```python
from build123d import *

# Parameters (mm, degrees)
SKETCH1_R           = 2.345368149
BOSS_EXTRUDE1_DEPTH = 8.89
SKETCH2_R           = 9.131634977
BOSS_EXTRUDE2_DEPTH = 10
SKETCH3_R           = 7.205640658
CUT_EXTRUDE1_DEPTH  = 2.54
FILLET1_R           = 2.54
FILLET2_R           = 2.54


# Some blends are built 0.0001 mm under size
with BuildPart() as part:
    # Sketch1 → Boss-Extrude1 (new body)
    with BuildSketch(Plane.XY):
        with Locations((21.750777604, -13.836740686)):
            Circle(SKETCH1_R)
    extrude(amount=BOSS_EXTRUDE1_DEPTH)

    # Sketch2 → Boss-Extrude2 (add)
    with BuildSketch(Plane.XY.offset(8.89)):
        with Locations((21.750777604, -13.836740686)):
            Circle(SKETCH2_R)
    extrude(amount=BOSS_EXTRUDE2_DEPTH)

    # Sketch3 → Cut-Extrude1 (cut)
    with BuildSketch(Plane.XY.offset(18.89)):
        with Locations((21.750777604, -13.836740686)):
            Circle(SKETCH3_R)
    extrude(amount=-CUT_EXTRUDE1_DEPTH, mode=Mode.SUBTRACT)

    # Fillet1
    fillet1_edges = [part.edges().sort_by_distance(p)[0] for p in [
        (14.545136946, -13.836740686, 16.35),
    ]]
    fillet(fillet1_edges, radius=FILLET1_R - 0.0001)  # a hair under: the kernel refuses the full size

    # Fillet2
    # the kernel refuses this fillet: 2.54 mm, written as the material it takes off along each edge
    with BuildSketch(Plane(origin=(21.750777604, -13.836740686, 8.89), x_dir=(1, 0, 0), z_dir=(0, -1, 0))) as fillet2_piece_1:
        with BuildLine():
            CenterArc((9.131634977 - FILLET2_R, FILLET2_R), FILLET2_R, 270, 90)
            Line((9.131634977 - FILLET2_R, 0), (9.131634977 - FILLET2_R, -FILLET2_R * 0.02))
            Line((9.131634977 - FILLET2_R, -FILLET2_R * 0.02), (9.131634977 + FILLET2_R * 0.02, -FILLET2_R * 0.02))
            Line((9.131634977 + FILLET2_R * 0.02, -FILLET2_R * 0.02), (9.131634977 + FILLET2_R * 0.02, FILLET2_R))
            Line((9.131634977 + FILLET2_R * 0.02, FILLET2_R), (9.131634977, FILLET2_R))
        make_face()
    revolve(axis=Axis((21.750777604, -13.836740686, 8.89), (0, 0, 1)), mode=Mode.SUBTRACT)
    with BuildSketch(Plane(origin=(21.750777604, -13.836740686, 18.89), x_dir=(1, 0, 0), z_dir=(0, -1, 0))) as fillet2_piece_2:
        with BuildLine():
            CenterArc((6.591634977, -2.46466976), FILLET2_R, 0, 76.011064225)
            Line((9.131634977, -2.46466976), (9.182434977, -2.46466976))
            Line((9.182434977, -2.46466976), (9.182434977, 0))
            Line((9.182434977, 0), (9.131634977, 0.0508))
            ThreePointArc((9.131634977, 0.0508), (8.168637817, 0.0508), (7.217920771, 0.049293395))
            Line((7.217920771, 0.049293395), (7.205640658, 0))
        make_face()
    revolve(axis=Axis((21.750777604, -13.836740686, 18.89), (0, 0, 1)), mode=Mode.SUBTRACT)


solid = part.part
```
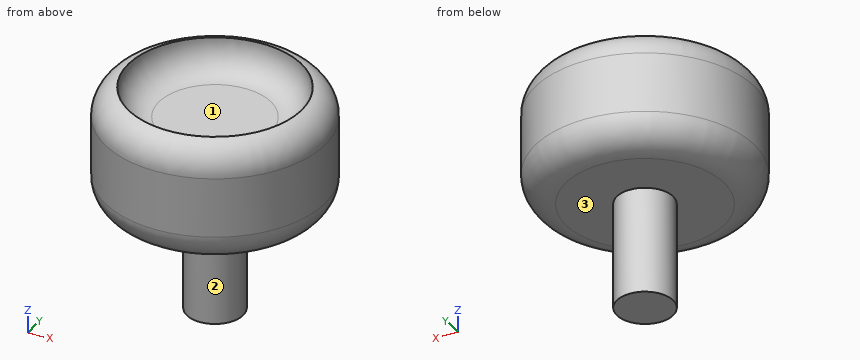
For this review, take the finished solid that the model builds, in its own axes (mm). Face numbers are marked on the shaded views. Round coordinates to 2 decimals unless told otherwise and drop trailing zeros. Write each loop counter-clockwise with the first axis right and the second up, starting at its lowest first coordinate (ties: lowest second). Pieces come first, ordered by that corner, then holes. Notation, with made-up numbers: (87, 73.25) - (94, 73.25) arc R23 ccw to (94, 99.25) - close; hole circle Ø7 at (-30.5, 18). An arc over 180 degrees is marked (long way). Answer as CSV lines item,"result". Start each with the question number.
(1) For line 1 (Z direction, x = 19, y = -15.75); line 2 (X direction, y = -17, z = 17.25); line 3 (X direction, y = -15.75, z = 17.5), list the stretches that pass through material, from the lowest coordinate up.
(2) Add section A-A, the plane z = 2. State the section outline as (x, y) points.
(3) Add section B-B, the plane z = 17.75. State the section outline as (x, y) points.
(4) Mouldability with a two-part tool opening along Y and no side actions: class the marked faces 1, 2 and 3 as +Y half, -Y half, draft (parallel to the pull), parting line (faces both ways), or undercut.
(5) For pin 1 (2 mm diameter, centred on x = 16.5, y = -16.5, fed in from +Z); pin 2 (3 mm diameter, centred on x = 26, y = -15, fed in from +Z); pin 3 (6 mm diameter, centred on y = -19, z = 7, fed in from -X), all flat-tipped, find the tip position at first contact; note any pin that passes through.
(6) Add section C-C, the plane z = 14.25. State the section outline as (x, y) points.
From the geometry:
1,line 1,"z = 8.89 to 16.35"
1,line 2,"x = 13.33 to 15.95, 27.55 to 30.17"
1,line 3,"x = 13.07 to 15.23, 28.27 to 30.44"
2,outline,"circle Ø4.69 at (21.75, -13.84)"
3,outline,"circle Ø17.52 at (21.75, -13.84); hole circle Ø13.87 at (21.75, -13.84)"
4,face 1,"undercut"
4,face 2,"parting line"
4,face 3,"draft"
5,pin 1,"stops at z = 17.66"
5,pin 2,"stops at z = 16.67"
5,pin 3,"stops at x = 14.23"
6,outline,"circle Ø18.26 at (21.75, -13.84)"
